Part model, mm, in its own coordinate system. Face numbers are marked on the shaded views. Round coordinates to 2 decimals unless told otherwise and drop trailing zeros. Write each loop counter-clockwise with the first axis right and the second up, starting at its lowest first coordinate (ties: lowest second). Pieces come first, ordered by that corner, then holes. Notation, with made-up numbers: M 72,10.25 L 98,10.25 A10 ccw 98,22.25 Z; hole C 75.25,46.5 d5. An arc over 180 degrees is marked long. Use one line per item in the form item = value. Start each with the question number.
Item 1: Cut at C-C, the plane x = 41.5. Give the cut face in (y, z), then the cut area to 3 significant figures.
Item 2: Probe L1, parallel to X at y = 80, z = 2.15; L2, parallel to Y at x = 0, z = 1.85; L3, parallel to X at y = 80, z = 4.4. List the from-to ranges inside material, lowest first.
Item 3: Cut at B-B, the plane y = 29. Give the cut face in (x, z), then the cut area to 4 significant figures.
Item 4: Mould opens along X. For the marked faces 1 and 2 say: +X half, -X half, draft (parallel to the pull), parting line (faces both ways), or undercut.
Item 5: Flat gauge pins, fed straight in: pin 1 Ø4.5 at (x, y) = (121.5, 80) entering from +Z; pin 2 Ø8 at (x, y) = (61, 8) entering from +Z. Where does each tip first touch, or does it go through?
Item 6: Cut at A-A, the plane z = 5.1. Give the cut face in (x, y).
Autodesk Fusion 360 part; units mm, degrees
sketch "Sketch1" plane through (0, 0, 0) normal (0, 0, 1) x (1, 0, 0)
  circle A0 centre (0, 0) radius 1.8
  circle A1 centre (121.5, 0) radius 1.8
  circle A2 centre (0, 80) radius 1.8
  circle A3 centre (121.5, 80) radius 1.8
  line L0 (-5, -5) -> (126.5, -5)
  line L1 (126.5, -5) -> (126.5, 85)
  line L2 (126.5, 85) -> (-5, 85)
  line L3 (-5, 85) -> (-5, -5)
  dimension "d3" = 121.5
  dimension "d4" = 80
  dimension "d5" = 3.6
  dimension "d6" = 5
  dimension "d7" = 5
  dimension "d8" = 5
  dimension "d9" = 5
extrude "Extrude1" add sketch "Sketch1" along normal blind 3
sketch "Sketch2" plane through (0, 0, 3) normal (0, 0, 1) x (-1, 0, 0)
  circle A0 centre (0, 0) radius 1.8
  circle A1 centre (0, -80) radius 1.8
  circle A2 centre (-121.5, 0) radius 1.8
  circle A3 centre (-121.5, -80) radius 1.8
  line L0 (5, -85) -> (5, 5)
  line L1 (5, 5) -> (-126.5, 5)
  line L2 (-126.5, 5) -> (-126.5, -85)
  line L3 (-126.5, -85) -> (5, -85)
  circle A4 centre (0, 0) radius 5
  line L4 (-5, 0) -> (-5, 5)
  line L5 (0, -5) -> (5, -5)
  circle A5 centre (-121.5, 0) radius 5
  line L6 (-116.5, 0) -> (-116.5, 5)
  line L7 (-121.5, -5) -> (-126.5, -5)
  circle A6 centre (-121.5, -80) radius 5
  line L8 (-116.5, -80) -> (-116.5, -85)
  line L9 (-121.5, -75) -> (-126.5, -75)
  circle A7 centre (0, -80) radius 5
  line L10 (-5, -80) -> (-5, -85)
  line L11 (0, -75) -> (5, -75)
extrude "Extrude2" add sketch "Sketch2" along normal blind 3 contours L0 L3 A7 | L0 A7 L11 | A7 | L3 A7 L10 | L0 A4 L5 | L3 A6 L8 | L0 L1 A4 | A4 | L2 L3 A6 | A6 | L1 A4 L4 | L2 A6 L9 | L1 A5 L6 | L2 A5 L7 | L1 L2 A5 | A5
equation "d7 = d6"
equation "d8 = d6"
equation "d9 = d6"
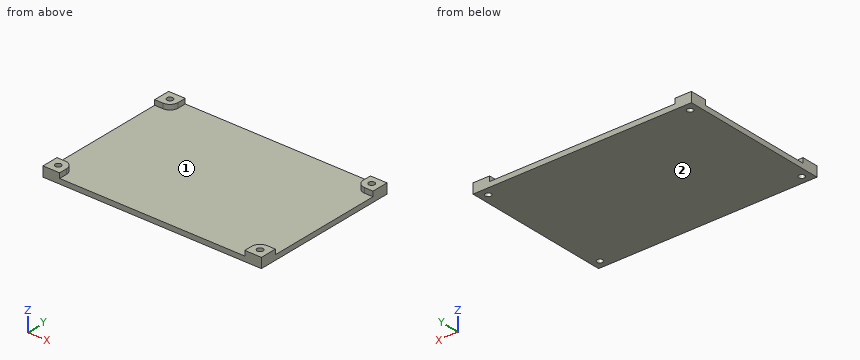
Model answer:
q1.outline = M -5,0 L 85,0 L 85,3 L -5,3 Z
q1.area = 270 mm²
q2.L1 = -5 to -1.8, 1.8 to 119.7, 123.3 to 126.5
q2.L2 = -5 to -1.8, 1.8 to 78.2, 81.8 to 85
q2.L3 = -5 to -1.8, 1.8 to 5, 116.5 to 119.7, 123.3 to 126.5
q3.outline = M -5,0 L 126.5,0 L 126.5,3 L -5,3 Z
q3.area = 394.5 mm²
q4.face_1 = undercut
q4.face_2 = draft
q5.pin_1 = 6
q5.pin_2 = 3
q6.outline = M -5,-5 L 5,-5 L 5,0 A5 ccw 0,5 L -5,5 Z; M -5,75 L 0,75 A5 ccw 5,80 L 5,85 L -5,85 Z; M 116.5,-5 L 126.5,-5 L 126.5,5 L 121.5,5 A5 ccw 116.5,0 Z; M 116.5,80 A5 ccw 121.5,75 L 126.5,75 L 126.5,85 L 116.5,85 Z; hole C 0,0 d3.6; hole C 0,80 d3.6; hole C 121.5,0 d3.6; hole C 121.5,80 d3.6
